CAD build for the part. Positions are in the model's coordinates, mm. Face numbers are marked on the shaded views. A direction names the side the tool comes from. Round coordinates to 2 decimals unless told otherwise and drop trailing zeros. Order: outer loops, then holes, each group sorted by start corner. A loop starts at its lowest first (then second) coordinate and runs counter-clockwise, first axis right, second up. Notation, with made-up numbers: M -39.5,30.25 L -11.5,30.25 A9 cw -11.5,47.25 Z; hole C 50,-5.5 d3. An arc over 180 degrees is marked long. Put each result on its own line as item: value.
Autodesk Inventor part; units mm, degrees
ref_plane "YZ Plane" through (0, 0, 0) normal (1, 0, 0) x (0, 1, 0)
ref_plane "XZ Plane" through (0, 0, 0) normal (0, 1, 0) x (-1, 0, 0)
ref_plane "XY Plane" through (0, 0, 0) normal (0, 0, 1) x (1, 0, 0)
sketch "Sketch1" plane through (0, 0, 0) normal (0, 1, 0) x (-1, 0, 0)
  line L0 (8, 8) -> (-8, 8)
  line L1 (-8, 8) -> (-8, -8)
  line L2 (-8, -8) -> (8, -8)
  line L3 (8, -8) -> (8, 8)
  line L4 (8, 8) -> (-8, -8) construction
  line L5 (-8, 8) -> (8, -8) construction
  point P0 (0, 0)
  dimension "d0" = 16
  dimension "d1" = 16
extrude "Extrusion1" add sketch "Sketch1" along normal blind 6.35
sketch "Sketch2" plane through (0, 6.35, 0) normal (0, 1, 0) x (1, 0, 0)
  line L0 (-8, 8) -> (-8, -8)
  line L1 (8, -8) -> (8, 8)
  point P0 (0, 0)
  point P1 (-4.825, 0)
  point P2 (4.825, 0)
hole "Hole1" at (-4.825, 6.35, 0) at (4.825, 6.35, 0) direction (0, -1, 0) diameter 2.1565 depth 4.29
sketch "Sketch3" plane through (8, 0, -8) normal (0, 0, -1) x (-1, 0, 0)
  point P0 (8, 0)
properties part number "bottom_cu_block" material "Copper"
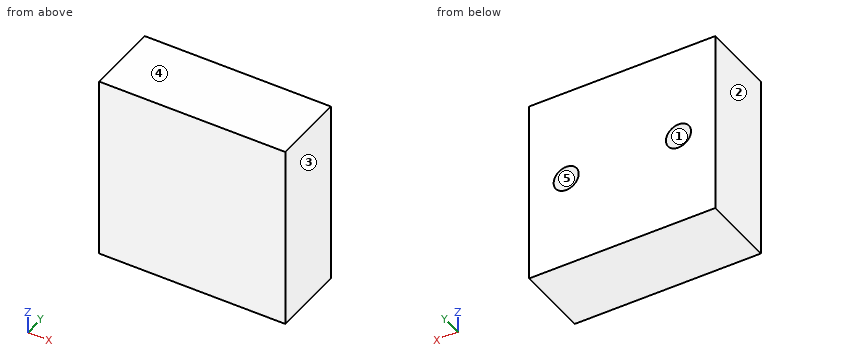
Item 1: Probe line 1 along X through (y, z) = (4.3, 0); line 2 along Z through (x, y) = (4.75, 4); line 3 along X through (y, z) = (2.5, 0.75). List the from-to ranges inside material, lowest first. Write a range as [from, to].
Answers below:
line 1: [-8, -5.9], [-3.75, 3.75], [5.9, 8]
line 2: [-8, -1.08], [1.08, 8]
line 3: [-8, -5.6], [-4.05, 4.05], [5.6, 8]
Item 2: Band-saw the part on C-C on x = -5.25. Give the cut face in (y, z).
Answers below:
outline: M 0,-8 L 6.35,-8 L 6.35,-0.99 L 2.06,-0.99 L 2.06,0.99 L 6.35,0.99 L 6.35,8 L 0,8 Z
Item 3: Mould opens along Z. For the marked faces 3, 4 and 5 say: pulls with the +Z half, pulls with the -Z half, needs draft (parallel to the pull), parting line crosses it, or undercut.
Answers below:
face 3: needs draft
face 4: pulls with the +Z half
face 5: undercut
Item 4: Band-saw the part on A-A on z = 0. Give the cut face in (x, y), and give its area (3 significant figures).
Answers below:
outline: M -8,0 L 8,0 L 8,6.35 L 5.9,6.35 L 5.9,2.06 L 3.75,2.06 L 3.75,6.35 L -3.75,6.35 L -3.75,2.06 L -5.9,2.06 L -5.9,6.35 L -8,6.35 Z
area: 83.1 mm²
Item 5: Band-saw the part on B-B on y = 4. Give the cut face in (x, z) (1 decimal), and give its area (3 significant figures).
Answers below:
outline: M -8,-8 L 8,-8 L 8,8 L -8,8 Z; hole C -4.8,0 d2.2; hole C 4.8,0 d2.2
area: 249 mm²
Item 6: Pin check, flat tip, straight feed: P1, Ø1.7, axis at x = -4.825, z = 0, coming from the +Y side. Stop position of the tip, or through.
Answers below:
P1: y = 2.06
Item 7: Tool access for the marked faces 1 and 2: list every direction of +Z, -Z, +X, -X, +Y, -Y with a clear straight run to the whole face (end or side of a thin tool).
Answers below:
face 1: +Y
face 2: +Z, -Z, -X, +Y, -Y
